from build123d import *

# Parameters (mm, degrees)
SKETCH1_R           = 1
BOSS_EXTRUDE1_DEPTH = 11
SKETCH2_R           = 2
BOSS_EXTRUDE2_DEPTH = 1.5
FILLET1_R           = 1


with BuildPart() as part:
    # Sketch1 → Boss-Extrude1 (new body)
    with BuildSketch(Plane(origin=(0, 0, 0), x_dir=(0, 0, -1), z_dir=(1, 0, 0))):
        Circle(SKETCH1_R)
    extrude(amount=BOSS_EXTRUDE1_DEPTH)

    # Sketch2 → Boss-Extrude2 (add)
    with BuildSketch(Plane.ZY):
        Circle(SKETCH2_R)
    extrude(amount=BOSS_EXTRUDE2_DEPTH)

    # Fillet1
    fillet1_edges = [part.edges().sort_by_distance(p)[0] for p in [
        (-1.5, 0, -2),
    ]]
    fillet(fillet1_edges, radius=FILLET1_R)


solid = part.part
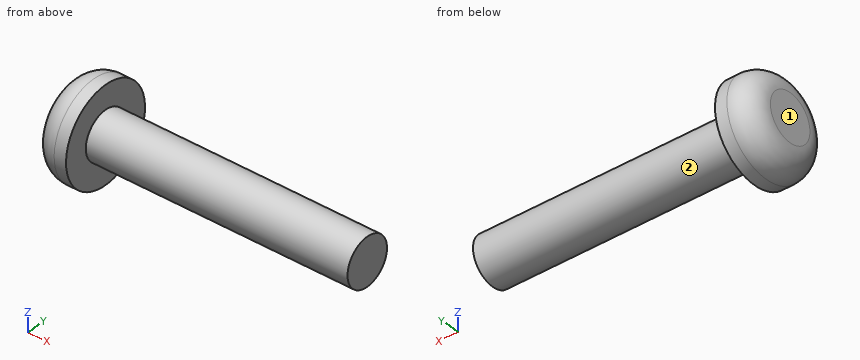
Geometry: final body of the model. Coordinates: model frame, mm. Face numbers are marked on the shaded views. A direction names the side the tool comes from. Coordinates: 2 decimals unless noted, no trailing zeros. Write each loop counter-clockwise with the first axis right and the second up, starting at its lowest first coordinate (ties: lowest second). Pieces come first, ordered by that corner, then holes. Notation, with made-up numbers: (-32.75, 53) - (-25.75, 53) arc R22 cw to (-25.75, 92) - close; hole circle Ø7 at (-12.75, 78.5). An arc over 180 degrees is marked (long way). Return JSON: item names as keys, results as strings.
Item 1: Reachability of the marked faces 1 and 2 from +Z, -Z, +X, -X, +Y, -Y: full face, straight path, thin tool, end or side. Return the list, or none.
Completed:
{"face 1": "+Z, -Z, -X, +Y, -Y", "face 2": "+X"}
Item 2: Section query A-A (x = 9). Output: boundary loops of the cut face in (y, z).
Completed:
{"outline": "circle Ø2 at (0, 0)"}
Item 3: Pin query (flat end, axial travel): pin 1 Ø1 at (x, z) = (3.5, 0) entering from -Y. Return the tip coordinate at first contact, or that it passes through.
Completed:
{"pin 1": "stops at y = -1"}
Item 4: Line query: L1, parallel to Z at x = 10.5, y = -0.05; L2, parallel to X at y = 1.2, z = -1.3; L3, parallel to Z at x = -1, y = 1.3. Output: solid intervals per line, ascending.
Completed:
{"L1": "z = -1 to 1", "L2": "x = -1.14 to 0", "L3": "z = -1.34 to 1.34"}
